Autodesk Inventor part; units mm, degrees
ref_plane "YZ Plane" through (0, 0, 0) normal (1, 0, 0) x (0, 1, 0)
ref_plane "XZ Plane" through (0, 0, 0) normal (0, 1, 0) x (-1, 0, 0)
ref_plane "XY Plane" through (0, 0, 0) normal (0, 0, 1) x (1, 0, 0)
sketch "Skizze1" plane through (0, 0, 0) normal (0, 0, 1) x (1, 0, 0)
  line L0 (-11.5, 11) -> (11.5, 11)
  line L1 (11.5, 11) -> (11.5, -11)
  line L2 (11.5, -11) -> (-11.5, -11)
  line L3 (-11.5, -11) -> (-11.5, 11)
  line L4 (0, -15.4) -> (0, 15.4)
  line L5 (-23.1, 0) -> (23.1, 0)
  line L6 (-11.5, 7) -> (-16.5, 7)
  line L7 (-16.5, 7) -> (-16.5, 5)
  line L8 (-16.5, 5) -> (-11.5, 5)
  line L9 (-11.5, 5) -> (-11.5, 7)
  line L10 (11.5, 7) -> (16.5, 7)
  line L11 (16.5, 7) -> (16.5, 5)
  line L12 (16.5, 5) -> (11.5, 5)
  line L13 (11.5, 5) -> (11.5, 7)
  point P0 (0, 0)
  dimension "d0" = 23
  dimension "d1" = 22
  dimension "d2" = 16
  dimension "d3" = 2
  dimension "d4" = 5
extrude "Extrusion1" add sketch "Skizze1" against normal mid plane 12 contours L0 L4 L5 L3 | L0 L1 L5 L4 | L5 L1 L2 L4 | L4 L2 L3 L5
extrude "Extrusion2" add sketch "Skizze1" along normal mid plane 12 contours L3 L8 L7 L6 | L10 L11 L12 L1
sketch "Skizze2" plane through (-11.5, 11, -6) normal (0, 1, 0) x (1, 0, 0)
  arc A0 (11.3431, -8) -> (11.3431, -4) centre (17, -6) ccw
  line L0 (0, 0) -> (23, 0)
  line L1 (23, 0) -> (23, -12)
  arc A1 (10.2601, -4) -> (10.2601, -8) centre (10.2601, -6) ccw
  line L2 (10.2601, -4) -> (11.3431, -4)
  line L3 (10.2601, -8) -> (11.3431, -8)
  point P0 (11.5, -6)
  dimension "d9" = 6
  dimension "d10" = 6
  dimension "d11" = 4
extrude "Extrusion3" add sketch "Skizze2" along normal blind 4 contours L3 A1 L2 A0
sketch "Skizze3" plane through (-16.5, 7, 6) normal (0, 1, 0) x (1, 0, 0)
  arc A0 (1.134, 5.5) -> (1.134, 6.5) centre (2, 6) ccw
  line L0 (0, 12) -> (0, 0)
  arc A1 (31.866, 6.5) -> (31.866, 5.5) centre (31, 6) ccw
  line L1 (33, 0) -> (33, 12)
  line L2 (1.134, 6.5) -> (0, 6.5)
  line L3 (1.134, 5.5) -> (0, 5.5)
  line L4 (31.866, 6.5) -> (33, 6.5)
  line L5 (33, 12) -> (33, 0)
  line L6 (31.866, 5.5) -> (33, 5.5)
  line L7 (-6.6, 6) -> (39.6, 6)
  line L8 (0, 6.5) -> (0, 5.5)
  line L9 (33, 6.5) -> (33, 5.5)
  point P0 (16.5, 6)
  dimension "d14" = 2
  dimension "d15" = 2
  dimension "d16" = 2
  dimension "d17" = 2
  dimension "d18" = 1
extrude "Extrusion4" cut sketch "Skizze3" against normal blind 2
sketch "Skizze4" plane through (-11.5, 15, -6) normal (0, 1, 0) x (1, 0, 0)
  circle A0 centre (17, -6) radius 2.25
  line L0 (23, -6) -> (23, -12)
  point P0 (11.5, -6)
  dimension "d21" = 4.5
  dimension "d22" = 6
extrude "Extrusion5" add sketch "Skizze4" along normal blind 3.5
properties part number "MicroServo"
Verification items for the finished model (mm, model axes). A direction names the side the tool comes from. Coordinates: 2 decimals unless noted, no trailing zeros. Loops run counter-clockwise (first coordinate to the right, second up) from the corner with the lowest first, then second, coordinate; pieces in that order, holes last. Notation, with made-up numbers: (-3, -20) -> (29, -20) arc R15 ccw to (29, -16) -> close; hole circle Ø2 at (45.5, -2.75). An arc over 180 degrees is marked (long way). Answer in a Markdown table with one row per item. Add a question column.
1. Access from +Z, -Z, +X, -X, +Y, -Y to the whole of each face (thin tool, end or side, straight path). Record for faces 4 (the face through (16, 6, -0.5)), 5 (the face through (-13, 7, 0)), 6 (the face through (-1, 13, -2)), 7 (the face through (-13, 5, 0)), 8 (the face through (10, 11, 5)).
2. Section check D-D, the plane x = -10.5. Enter the section's corners in (y, z).
3. Section check A-A, the plane x = 14.5. Enter the section's corners in (y, z).
4. Draft check along X on faces 1 (the face through (-13.5, 6, 0)), 2 (the face through (11.5, -3, 0)), 3 (the face through (-1, 13, 2)). Enter one of: +X half, -X half, draft (parallel to the pull), parting line (faces both ways), or undercut.
5. Section check C-C, the plane y = 11.5. Enter the section's corners in (x, z).
6. Section check B-B, the plane z = -3.5. Enter the section's corners in (x, y), then the cut area to 3 significant figures.
7. Depth check by flat-ended pin: P1, Ø1.2, axis at x = -0.5, y = 13.5, coming from the +Z side; P2, Ø2.5, axis at x = -14.5, z = 0, coming from the -Y side; P3, Ø2, axis at x = 1, z = -3.5, coming from the +Y side. Enter the tip coordinate at first touch or a pass-through.
8. Material ranges on probe 1 along Z at (x, y) = (-14.5, 6.15); probe 2 along X at (y, z) = (-5.75, -4); probe 3 along Y at (x, z) = (10, 0.75), recorded low to high. Write a range as [from, to].
Derived:
| question | item | result |
|---|---|---|
| 1 | face 4 | +X, +Y, -Y |
| 1 | face 5 | +Z, -Z, -X, +Y |
| 1 | face 6 | -Z, -X, +Y |
| 1 | face 7 | +Z, -Z, -X, -Y |
| 1 | face 8 | +Z, +X, +Y |
| 2 | outline | (-11, -6) -> (11, -6) -> (11, 6) -> (-11, 6) -> close |
| 3 | outline | (5, -6) -> (7, -6) -> (7, -1) -> (5, -1) -> close; (5, 1) -> (7, 1) -> (7, 6) -> (5, 6) -> close |
| 4 | face 1 | undercut |
| 4 | face 2 | +X half |
| 4 | face 3 | draft |
| 5 | outline | (-1.24, -2) -> (-0.16, -2) arc R6 ccw (long way) to (-0.16, 2) -> (-1.24, 2) arc R2 ccw to start |
| 6 | outline | (-16.5, 5) -> (-11.5, 5) -> (-11.5, -11) -> (11.5, -11) -> (11.5, 5) -> (16.5, 5) -> (16.5, 7) -> (11.5, 7) -> (11.5, 11) -> (10.37, 11) -> (10.37, 15) -> (0.63, 15) -> (0.63, 11) -> (-11.5, 11) -> (-11.5, 7) -> (-16.5, 7) -> close |
| 6 | area | 565 mm² |
| 7 | P1 | stops at z = 2.62 |
| 7 | P2 | stops at y = 5 |
| 7 | P3 | stops at y = 15 |
| 8 | probe 1 | z = [-6, -1], [1, 6] |
| 8 | probe 2 | x = [-11.5, 11.5] |
| 8 | probe 3 | y = [-11, 15] |
